Read the model definition and answer for the solid it produces. Units are mm, in the model's axes. Face numbers are marked on the shaded views. A direction names the side the tool comes from. Coordinates: 2 decimals unless noted, no trailing zeros. Loops run counter-clockwise (first coordinate to the right, second up) from the corner with the lowest first, then second, coordinate; pieces in that order, holes last. Notation, with made-up numbers: M -30,34.25 L 29,34.25 A13 ccw 29,51.25 Z; hole C 72.25,54.5 d8. An arc over 180 degrees is marked long. One line per item, written item: value. Start each with the question number.
1. Flat-ended cylindrical pins translate along their axes: pin 1 (0.9 mm diameter, centred on x = 0, y = 11.5, fed in from -Z); pin 2 (1.5 mm diameter, centred on x = 1, y = 11.5, fed in from +Z); pin 3 (4 mm diameter, centred on x = 2, y = 3, fed in from -Z). Find the tip coordinate at first contact, or state that the pin passes through.
2. The part is cut by section B-B (z = 0). Write down the section's boundary in (x, y), then the cut area to 4 significant figures.
3. For the marked faces 1 and 2, determine the directions among +Z, -Z, +X, -X, +Y, -Y from which every point of the face is accessible in a straight line to the end or side of a thin tool.
4. The part is cut by section A-A (y = 11.5). Write down the section's boundary in (x, z), then the cut area to 3 significant figures.
5. Determine the mould class of the marked faces 3, 4, 5 and 6 for opening direction Z: +Z half, -Z half, draft (parallel to the pull), parting line (faces both ways), or undercut.
6. The part is cut by section D-D (y = 21). Write down the section's boundary in (x, z), then the cut area to 3 significant figures.
7. Consider probe 1 along Y at (x, z) = (-2.75, -0.75); probe 2 along Y at (x, z) = (0, -4.35); probe 3 along Y at (x, z) = (0, -4.45). Determine where each line is inside the solid, lowest interval first.
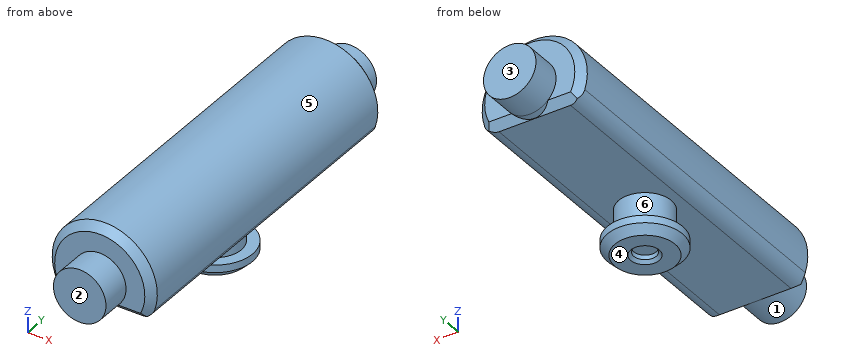
```python
from build123d import *

# Parameters (mm, degrees)
EXTRUDE_1_DEPTH     = 23
SKETCH_2_R          = 1.75
EXTRUDE_2_DEPTH     = 2
EXTRUDE_START       = 2
SKETCH_3_R          = 1.75
EXTRUDE_3_DEPTH     = 2
SKETCH_4_R          = 1.75
EXTRUDE_4_DEPTH     = 2
SKETCH_5_R          = 2.5
EXTRUDE_5_DEPTH     = 1
CHAMFER_1_SIZE      = 0.5
SKETCH_6_R          = 0.75
CUT_EXTRUDE_1_DEPTH = 0.5
CHAMFER_2_SIZE      = 0.2
CHAMFER_3_SIZE      = 0.5
FILLET_3_R          = 1


with BuildPart() as part:
    # 草图1 → 凸台-拉伸1 (new body)
    with BuildSketch(Plane(origin=(0, 0, 0), x_dir=(1, 0, 0), z_dir=(0, 1, 0))):
        with BuildLine():
            Line((-3.024810761, 1.76082931), (3.024810761, 1.76082931))
            ThreePointArc((3.024810761, 1.76082931), (0, -3.5), (-3.024810761, 1.76082931))
        make_face()
    extrude(amount=EXTRUDE_1_DEPTH)

    # 草图2 → 凸台-拉伸2 (add)
    with BuildSketch(Plane(origin=(0, 23, 0), x_dir=(1, 0, 0), z_dir=(0, 1, 0))):
        with Locations(Location((0, 0, 0), (0, 0, 270))):
            Circle(SKETCH_2_R)
    extrude(amount=EXTRUDE_2_DEPTH)

    # 草图3 → 凸台-拉伸3 (add)
    with BuildSketch(Plane.XZ.offset(EXTRUDE_START)):
        with Locations(Location((0, 0, 0), (0, 0, 90))):
            Circle(SKETCH_3_R)
    extrude(amount=-EXTRUDE_3_DEPTH)

    # 草图4 → 凸台-拉伸4 (add)
    with BuildSketch(Plane(origin=(0, 0, -1.76082931), x_dir=(-1, 0, 0), z_dir=(0, 0, -1))):
        with Locations(Location((0, 11.5, 0), (0, 0, 180))):
            Circle(SKETCH_4_R)
    extrude(amount=EXTRUDE_4_DEPTH)

    # 草图5 → 凸台-拉伸5 (add)
    with BuildSketch(Plane(origin=(0, 0, -3.76082931), x_dir=(-1, 0, 0), z_dir=(0, 0, -1))):
        with Locations((0, 11.5)):
            Circle(SKETCH_5_R)
    extrude(amount=EXTRUDE_5_DEPTH)

    # 倒角1
    chamfer_1_edges = [part.edges().sort_by_distance(p)[0] for p in [
        (2.5, 11.5, -4.76082931),
    ]]
    chamfer(chamfer_1_edges, length=CHAMFER_1_SIZE)

    # 草图6 → 切除-拉伸1 (cut)
    with BuildSketch(Plane(origin=(0, 0, -4.76082931), x_dir=(-1, 0, 0), z_dir=(0, 0, -1))):
        with Locations((0, 11.5)):
            Circle(SKETCH_6_R)
    extrude(amount=-CUT_EXTRUDE_1_DEPTH, mode=Mode.SUBTRACT)

    # 倒角2
    chamfer_2_edges = [part.edges().sort_by_distance(p)[0] for p in [
        (0.75, 11.5, -4.76082931),
    ]]
    chamfer(chamfer_2_edges, length=CHAMFER_2_SIZE)

    # 倒角3
    # the kernel refuses this chamfer: 0.5 mm, written as the material it takes off along each edge
    with BuildSketch(Plane(origin=(-4.310652255, 0, -1.76082931), x_dir=(0, 0.9996219169112968, -0.027495876610586494), z_dir=(1, 0, 0))) as chamfer_3_piece_1_section:
        Polygon((CHAMFER_3_SIZE * 0.999621916911, CHAMFER_3_SIZE * 0.0274958766106), (-CHAMFER_3_SIZE * 0.0274958766106, CHAMFER_3_SIZE * 0.999621916911), (0, 0), align=None)
    chamfer_3_piece_1 = extrude(amount=8.62130451, mode=Mode.PRIVATE)
    chamfer_3_piece_1 = chamfer_3_piece_1 - Plane(origin=(0, 0.410648891, 0), x_dir=(0, 0, 1), z_dir=(0, -1, 0)) * Cylinder(1.75, 20, mode=Mode.PRIVATE)
    add(chamfer_3_piece_1, mode=Mode.SUBTRACT)
    with BuildSketch(Plane(origin=(0, 0, 0), x_dir=(0.625040137107155, 0, -0.7805926127020859), z_dir=(-0.7805926127020859, 0, -0.625040137107155))) as chamfer_3_piece_2:
        Polygon((3.5, -CHAMFER_3_SIZE), (3.5 - CHAMFER_3_SIZE, 0), (3.5, 0), align=None)
    revolve(axis=Axis((0, 0, 0), (0, -1, 0)), revolution_arc=282.629733058, mode=Mode.SUBTRACT)
    with BuildSketch(Plane(origin=(0, 23, 0), x_dir=(0.6250401371071543, 0, -0.7805926127020866), z_dir=(-0.7805926127020866, 0, -0.6250401371071543))) as chamfer_3_piece_3:
        Polygon((3.5, CHAMFER_3_SIZE), (3.5 - CHAMFER_3_SIZE, 0), (3.5, 0), align=None)
    revolve(axis=Axis((0, 23, 0), (0, -1, 0)), revolution_arc=282.629733058, mode=Mode.SUBTRACT)
    with BuildSketch(Plane(origin=(-4.310652255, 23, -1.76082931), x_dir=(0, -0.9996219169112968, -0.027495876610586414), z_dir=(1, 0, 0))) as chamfer_3_piece_4_section:
        Polygon((CHAMFER_3_SIZE * 0.999621916911, -CHAMFER_3_SIZE * 0.0274958766106), (-CHAMFER_3_SIZE * 0.0274958766106, -CHAMFER_3_SIZE * 0.999621916911), (0, 0), align=None)
    chamfer_3_piece_4 = extrude(amount=8.62130451, mode=Mode.PRIVATE)
    chamfer_3_piece_4 = chamfer_3_piece_4 - Plane(origin=(0, 22.589351109, 0), x_dir=(0, 0, 1), z_dir=(0, -1, 0)) * Cylinder(1.75, 20, mode=Mode.PRIVATE)
    add(chamfer_3_piece_4, mode=Mode.SUBTRACT)

    # 圆角3
    fillet_3_edges = [part.edges().sort_by_distance(p)[0] for p in [
        (3.024810761, 11.5, -1.76082931),
        (-3.024810761, 11.5, -1.76082931),
    ]]
    fillet(fillet_3_edges, radius=FILLET_3_R)


solid = part.part
```
Answer block:
1. pin 1: stops at z = -4.26
1. pin 2: stops at z = 3.49
1. pin 3: stops at z = -1.76
2. outline: M -3.5,0.5 L -3,0 L -1.75,0 L -1.75,-2 L 1.75,-2 L 1.75,0 L 3,0 L 3.5,0.5 L 3.5,22.5 L 3,23 L 1.75,23 L 1.75,25 L -1.75,25 L -1.75,23 L -3,23 L -3.5,22.5 Z
2. area: 174.5 mm2
3. face 1: -Y
3. face 2: +Z, -Z, +X, -X, -Y
4. outline: M -3.33,-1.07 A1 ccw -2.38,-1.76 L -1.75,-1.76 L -1.75,-3.76 L -2.5,-3.76 L -2.5,-4.26 L -2,-4.76 L -0.95,-4.76 L -0.75,-4.56 L -0.75,-4.26 L 0.75,-4.26 L 0.75,-4.56 L 0.95,-4.76 L 2,-4.76 L 2.5,-4.26 L 2.5,-3.76 L 1.75,-3.76 L 1.75,-1.76 L 2.38,-1.76 A1 ccw 3.33,-1.07 A3.5 ccw long Z
4. area: 41.8 mm2
5. face 3: draft
5. face 4: -Z half
5. face 5: parting line
5. face 6: undercut
6. outline: M -3.33,-1.07 A1 ccw -2.38,-1.76 L 2.38,-1.76 A1 ccw 3.33,-1.07 A3.5 ccw long Z
6. area: 30.9 mm2
7. probe 1: y = 0 to 23
7. probe 2: y = 9.09 to 10.75, 12.25 to 13.91
7. probe 3: y = 9.19 to 10.75, 12.25 to 13.81
